from build123d import *

# Parameters (mm, degrees)
SKETCH_1_R      = 0.4
EXTRUDE_1_DEPTH = 10
SKETCH_2_W      = 80
SKETCH_2_H      = 0.8
EXTRUDE_2_DEPTH = 0.8
FILLET_1_R      = 0.4
SKETCH_3_R      = 0.4
EXTRUDE_3_DEPTH = 3.2
SKETCH_4_R      = 0.4
EXTRUDE_4_DEPTH = 3.2


with BuildPart() as part:
    # 草图1 → 凸台-拉伸1 (new body)
    with BuildSketch(Plane(origin=(0, 0, 0), x_dir=(1, 0, 0), z_dir=(0, 1, 0))):
        with Locations(Location((0, 0, 0), (0, 0, 270))):
            Circle(SKETCH_1_R)
    extrude(amount=EXTRUDE_1_DEPTH)

    # 草图2 → 凸台-拉伸2 (add)
    with BuildSketch(Plane(origin=(0, 10, 0), x_dir=(1, 0, 0), z_dir=(0, 1, 0))):
        Rectangle(SKETCH_2_W, SKETCH_2_H)
    extrude(amount=EXTRUDE_2_DEPTH)

    # 圆角1
    fillet_1_edges = [part.edges().sort_by_distance(p)[0] for p in [
        (40, 10, 0),
        (40, 10.8, 0),
        (-40, 10, 0),
        (-40, 10.8, 0),
    ]]
    fillet(fillet_1_edges, radius=FILLET_1_R - 0.0001)  # a hair under: the kernel refuses the full size

    # 草图3 → 凸台-拉伸3 (add)
    with BuildSketch(Plane.XY.offset(0.4)):
        with Locations((39.6, 10.4)):
            Circle(SKETCH_3_R)
    extrude(amount=EXTRUDE_3_DEPTH)

    # 草图4 → 凸台-拉伸4 (add)
    with BuildSketch(Plane(origin=(0, 0, -0.4), x_dir=(-1, 0, 0), z_dir=(0, 0, -1))):
        with Locations((39.6, 10.4)):
            Circle(SKETCH_4_R)
    extrude(amount=EXTRUDE_4_DEPTH)

    # 草图5 → 旋转1 (revolve)
    with BuildSketch(Plane(origin=(0, 10.4, 0), x_dir=(1, 0, 0), z_dir=(0, 1, 0))):
        Polygon((39.6, -3.6), (39.6, -5.4), (40, -3.6), align=None)
    revolve(axis=Axis((39.6, 10.4, 3.6), (0, 0, 1)))

    # 草图6 → 旋转2 (revolve)
    with BuildSketch(Plane(origin=(0, 10.4, 0), x_dir=(1, 0, 0), z_dir=(0, 1, 0))):
        Polygon((-39.6, 3.6), (-39.6, 5.4), (-40, 3.6), align=None)
    revolve(axis=Axis((-39.6, 10.4, -3.6), (0, 0, -1)))


solid = part.part
Verification items for the finished model (mm, model axes). Round coordinates to 2 decimals unless told otherwise and drop trailing zeros. Loops run counter-clockwise (first coordinate to the right, second up) from the corner with the lowest first, then second, coordinate; pieces in that order, holes last. Notation, with made-up numbers: (75, 44) - (103, 44) arc R19 ccw to (103, 78) - close; hole circle Ø11 at (-28, 23.5). An arc over 180 degrees is marked (long way). Answer in a Markdown table with one row per item. Add a question column.
Q1. Material ranges on line 1 (Y direction, x = 34, z = 0), recorded low to high.
Q2. Section check A-A on y = 5.75. Enter the section's corners in (x, z).
Q3. Gauge pin test, flat ends, axial feed: pin 1 (0.9 mm diameter, centred on x = 15.5, z = 0, fed in from -Y); pin 2 (1.5 mm diameter, centred on x = -18.5, y = 7.5, fed in from -Z); pin 3 (0.6 mm diameter, centred on x = 18, y = 10.5, fed in from +Z); pin 4 (1.5 mm diameter, centred on y = 9, z = 0.5, fed in from -X). Record the tip position at first contact, or that the pin passes through.
Q4. Section check C-C on x = 19. Enter the section's corners in (y, z).
Q5. Section check B-B on z = 1.5. Enter the section's corners in (x, y).
Found:
| question | item | result |
|---|---|---|
| 1 | line 1 | y = 10 to 10.8 |
| 2 | outline | circle Ø0.8 at (0, 0) |
| 3 | pin 1 | stops at y = 10 |
| 3 | pin 2 | passes through |
| 3 | pin 3 | stops at z = 0.4 |
| 3 | pin 4 | stops at x = -0.4 |
| 4 | outline | (10, -0.4) - (10.8, -0.4) - (10.8, 0.4) - (10, 0.4) - close |
| 5 | outline | circle Ø0.8 at (39.6, 10.4) |
